Could you check a few things on this model? Use its own coordinates, in mm. Face numbers are marked on the shaded views. A direction names the side the tool comes from. Round coordinates to 2 decimals unless told otherwise and drop trailing zeros. Loops run counter-clockwise (first coordinate to the right, second up) from the corner with the lowest first, then second, coordinate; pieces in that order, holes last.
from build123d import *

# Parameters (mm, degrees)
BOSS_EXTRUDE1_DEPTH = 15
SKETCH2_R           = 2.6
CUT_EXTRUDE1_DEPTH  = 56.235857919
SKETCH3_R           = 1.5
CUT_EXTRUDE2_DEPTH  = 52.874849397
FILLET1_R           = 7.5


with BuildPart() as part:
    # Sketch1 → Boss-Extrude1 (new body)
    with BuildSketch(Plane(origin=(0, 0, 0), x_dir=(0, 0, -1), z_dir=(1, 0, 0))):
        Polygon((0, 0), (51, 0), (51, 3.916666667), (51, 21), (45, 21), (45, 6), (0, 6), align=None)
    extrude(amount=BOSS_EXTRUDE1_DEPTH)

    # Sketch2 → Cut-Extrude1 (cut, through all)
    with BuildSketch(Plane(origin=(0, 6, 0), x_dir=(1, 0, 0), z_dir=(0, 1, 0))):
        with Locations(Location((7.5, 7, 0), (0, 0, 270))):
            Circle(SKETCH2_R)
    extrude(amount=-CUT_EXTRUDE1_DEPTH, mode=Mode.SUBTRACT)

    # Sketch3 → Cut-Extrude2 (cut, through all)
    with BuildSketch(Plane.XY.offset(-45)):
        with Locations((7.5, 13.5)):
            Circle(SKETCH3_R)
    extrude(amount=-CUT_EXTRUDE2_DEPTH, mode=Mode.SUBTRACT)

    # Fillet1
    fillet1_edges = [part.edges().sort_by_distance(p)[0] for p in [
        (0, 21, -48),
        (15, 21, -48),
    ]]
    fillet(fillet1_edges, radius=FILLET1_R - 0.0001)  # a hair under: the kernel refuses the full size


solid = part.part
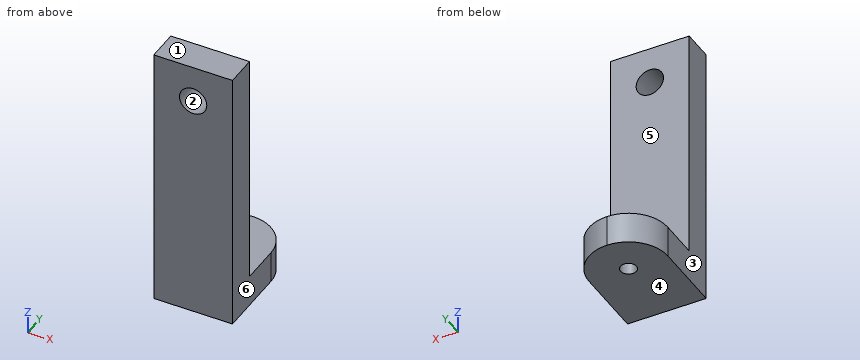
Item 1: For the marked faces 5 and 6, which set-ups out of +Z, -Z, +X, -X, +Y, -Y let a thin tool reach every point of the face, with its end or its side?
Results list:
face 5: +Z, +X, -X, +Y
face 6: +Z, -Z, +X, +Y, -Y
Item 2: If we section it at A-A, the plane z = -7: Please give me the cut outline in (x, y).
Results list:
outline: (0, 0) - (4.9, 0) - (4.9, 6) - (0, 6) - close; (10.1, 0) - (15, 0) - (15, 6) - (10.1, 6) - close
Item 3: If we section it at B-B, the plane y = 12.75: Please give me the cut outline in (x, z).
Results list:
outline: (0, -51) - (6.2, -51) - (6.2, -45) - (0, -45) - close; (8.8, -51) - (15, -51) - (15, -45) - (8.8, -45) - close
Item 4: Will these pins go through, and if not, where does the flat tip stop? pin 1 (8 mm diameter, centred on y = 6, z = -42.5, fed in from -X); pin 2 (1 mm diameter, centred on x = 11, y = 8.5, fed in from +Z); pin 3 (4.5 mm diameter, centred on x = 7, z = -26, fed in from +Y); pin 4 (1.5 mm diameter, centred on y = 14.5, z = -43, fed in from -X).
Results list:
pin 1: stops at x = 0
pin 2: stops at z = -45
pin 3: stops at y = 6
pin 4: passes through
Item 5: If I drill on line 1 along Y through (x, z) = (7.5, -48.8); line 2 along X through (y, z) = (3.4, -7); line 3 along Z through (x, y) = (1, 13), over which ranges is the centre line in solid material (lowest first)?
Results list:
line 1: y = 0 to 12, 15 to 21
line 2: x = 0 to 4.9, 10.1 to 15
line 3: z = -51 to -45
Item 6: If we section it at D-D, the plane z = -13.5: Please give me the cut outline in (x, y), then the cut area to 3 significant figures.
Results list:
outline: (0, 0) - (15, 0) - (15, 6) - (0, 6) - close
area: 90.0 mm2
Item 7: We'd pull the mould along Z, two halves only. Please class the marked faces 1, 2, 3 and 4: released by +Z, released by -Z, zero draft, split by the parting line, or undercut.
Results list:
face 1: released by +Z
face 2: undercut
face 3: zero draft
face 4: released by -Z
Item 8: If we section it at C-C, the plane x = 3.5: Please give me the cut outline in (y, z).
Results list:
outline: (0, -51) - (19.84, -51) - (19.84, -45) - (6, -45) - (6, 0) - (0, 0) - close
